from build123d import *

# Parameters (mm, degrees)
PAD_DEPTH       = 15
SKETCH002_R     = 67
POCKET_DEPTH    = 13.5
POCKET001_DEPTH = 13.5
PAD001_DEPTH    = 35
PAD002_DEPTH    = 35
SKETCH_R        = 9.5
POCKET002_DEPTH = 45.1514534441
SKETCH007_R     = 9.5
POCKET003_DEPTH = 93.6873432021


with BuildPart() as part:
    # Sketch001 → Pad (new body)
    with BuildSketch(Plane.XY):
        with BuildLine():
            ThreePointArc((71.2460525222, 20), (44.7436533058, 58.9406946756), (0.1121090023, 73.9999150781))
            Line((0.1121090023, 73.9999150781), (-70, 74.1061334774))
            ThreePointArc((-69.9999999999, 74.1061334774), (-89.3215614177, 42.9266570301), (-52.7907882568, 39.6122793491))
            ThreePointArc((63.5437766663, 17.8378375087), (12.1424161228, 64.8734285413), (-52.7907882568, 39.6122793491))
            ThreePointArc((63.5437766663, 17.8378375087), (68.4759958054, 15.0677809492), (71.2460525222, 20))
        make_face()
    extrude(amount=PAD_DEPTH)

    # Sketch002 → Pocket (cut)
    with BuildSketch(Plane(origin=(0, 0, 0), x_dir=(1, 0, 0), z_dir=(0, 0, -1))):
        Circle(SKETCH002_R)
    extrude(amount=-POCKET_DEPTH, mode=Mode.SUBTRACT)

    # Sketch003 → Pocket001 (cut)
    with BuildSketch(Plane(origin=(0, 0, 0), x_dir=(1, 0, 0), z_dir=(0, 0, -1))):
        Polygon((-153.2553251378, -67.2322555451), (0.1014988729, -66.9999231192), (-35.4631, 35.7409), align=None)
    extrude(amount=-POCKET001_DEPTH, mode=Mode.SUBTRACT)

    # Sketch005 → Pad001 (new body)
    with BuildSketch(Plane.XY.offset(15)):
        Polygon((35.7520138156, 58.6156421796), (42.6985975202, 65.809040183), (64.2787915304, 44.9692890692), (57.3322078258, 37.7758910658), align=None)
    extrude(amount=-PAD001_DEPTH)

    # Sketch006 → Pad002 (new body)
    with BuildSketch(Plane.XY.offset(15)):
        Polygon((-41.8276469497, 71.0634495008), (-43.8797678097, 76.7016052255), (-15.6889891861, 86.9622095253), (-9.8847001983, 71.0150565952), align=None)
    extrude(amount=-PAD002_DEPTH)

    # Sketch → Pocket002 (cut, through all)
    with BuildSketch(Plane(origin=(46.5421108207, 48.1957666227, 0), x_dir=(0.7193398003, -0.6946583705, 0), z_dir=(-0.6946583705, -0.7193398003, 0))):
        with Locations((0, -20)):
            Circle(SKETCH_R)
    extrude(amount=-POCKET002_DEPTH, mode=Mode.SUBTRACT)

    # Sketch007 → Pocket003 (cut, through all)
    with BuildSketch(Plane(origin=(-28.4858461346, 78.2642190287, 0), x_dir=(-0.9396926208, -0.3420201433, 0), z_dir=(-0.3420201433, 0.9396926208, 0))):
        with Locations((0, -20)):
            Circle(SKETCH007_R)
    extrude(amount=-POCKET003_DEPTH, mode=Mode.SUBTRACT)


solid = part.part
Work out the finished part from the listing and answer in its coordinate system (mm). A direction names the side the tool comes from. Give positions to 0.01 mm unless a question says otherwise; leave off trailing zeros. Loops run counter-clockwise (first coordinate to the right, second up) from the corner with the lowest first, then second, coordinate; pieces in that order, holes last. Notation, with made-up numbers: (19, 59) - (76, 59) arc R29 cw to (76, 97) - close; hole circle Ø1 at (10, -36.5). An arc over 180 degrees is marked (long way). Answer in a Markdown table with one row per item.
(1) For a pull along Y with two mould halves and no side action, classify faces 1 (the face through (50.1, 51.6, -10.5)), 2 (the face through (13.151, 64.677, 14.24)), 3 (the face through (-83.374, 69.482, 9.132)) as pulls with the +Y half, pulls with the -Y half, needs draft (parallel to the pull), parting line crosses it, or undercut.
Results list:
| item | result |
|---|---|
| face 1 | undercut |
| face 2 | pulls with the -Y half |
| face 3 | parting line crosses it |
(2) A tool of negligible diameter and unlimited length cuts with its end or side. For faces 4 (the face through (46.693, 48.05, -7.638)), 5 (the face through (-28.36, 78.31, -16.24)), 6 (the face through (61.626, 42.222, -6.144)), from which of +Z, -Z, +X, -X, +Y, -Y can it reach the whole face along a straight path? Write none if from no direction.
Results list:
| item | result |
|---|---|
| face 4 | -Z, -X, -Y |
| face 5 | -Z |
| face 6 | -Z, +X |
(3) Section C-C (z = 1.5) is taken. Give the vertices of the cut face in (x, y), and give its area (3 significant figures).
Results list:
| item | result |
|---|---|
| outline | (-85.91, 67.13) - (0.1, 67) arc R67 cw to (65.16, 15.6) arc R4 ccw to (71.25, 20) arc R74 ccw to (61.13, 41.71) - (64.28, 44.97) - (42.7, 65.81) - (39.55, 62.55) arc R74 ccw to (0.11, 74) - (-10.98, 74.02) - (-15.69, 86.96) - (-43.88, 76.7) - (-42.92, 74.07) - (-70, 74.11) arc R21.56 ccw to start |
| area | 1,580 mm² |
(4) Section D-D (x = -56) is taken. Give the vertices of the cut face in (y, z).
Results list:
| item | result |
|---|---|
| outline | (36.19, 13.5) - (67.08, 13.5) - (67.08, 0) - (74.08, 0) - (74.08, 15) - (36.19, 15) - close |
(5) Flat-ended cylindrical pins translate along their axes: pin 1 Ø5 at (y, z) = (35.5, -5) entering from -X; pin 2 Ø10 at (x, z) = (-58, -3.5) entering from +Y; pin 3 Ø10 at (x, y) = (21.5, 68.5) entering from -Z. Find the tip coordinate at first contact, or state that the pin passes through.
Results list:
| item | result |
|---|---|
| pin 1 | stops at x = 57.1 |
| pin 2 | stops at y = 74.09 |
| pin 3 | stops at z = 0 |
(6) Section B-B (z = -17.5) is taken. Give the vertices of the cut face in (x, y), and give its area (3 significant figures).
Results list:
| item | result |
|---|---|
| outline | (-43.88, 76.7) - (-41.83, 71.06) - (-35.61, 71.05) - (-37.1, 75.13) - (-19.87, 81.4) - (-16.1, 71.02) - (-9.88, 71.02) - (-15.69, 86.96) - close; (35.75, 58.62) - (39.95, 54.56) - (46.9, 61.76) - (42.7, 65.81) - close; (53.13, 41.83) - (57.33, 37.78) - (64.28, 44.97) - (60.08, 49.02) - close |
| area | 320 mm² |
(7) Section A-A (z = -6.5) is taken. Give the vertices of the cut face in (x, y).
Results list:
| item | result |
|---|---|
| outline | (-43.88, 76.7) - (-41.83, 71.06) - (-9.88, 71.02) - (-15.69, 86.96) - close; (35.75, 58.62) - (57.33, 37.78) - (64.28, 44.97) - (42.7, 65.81) - close |
(8) Consider L1, parallel to Z at x = -77, y = 66; L2, parallel to X at y = 71.5, z = -14; L3, parallel to X at y = 51.5, z = -2.5. Determine where each line is inside the solid, lowest interval first. Write a range as [from, to].
Results list:
| item | result |
|---|---|
| L1 | z = [13.5, 15] |
| L2 | x = [-41.99, -33.86], [-18.19, -10.06] |
| L3 | x = [43.12, 57.52] |
